Source: CAD feature listing. Evaluate the final solid. Frame: model axes, mm. A direction names the side the tool comes from. Give positions to 0.01 mm unless a question says otherwise; leave off trailing zeros. Write each loop counter-clockwise with the first axis right and the second up, starting at its lowest first coordinate (ties: lowest second). Pieces come first, ordered by that corner, then holes. Notation, with made-up numbers: (49, 43) -> (85, 43) arc R3 ccw to (85, 47) -> close; hole circle Ø11 at (42.5, -1). An arc over 180 degrees is marked (long way). Use one line per item in the form item = value. Start each with the question number.
(1) Cut plane C-C, the plane z = -12. Output: boundary loops of the cut face in (x, y).
(2) Draft query along Y for faces 1 (the face through (0, 6, 2)), 2 (the face through (-22, -0.1, 4.5)), 3 (the face through (-3.233, -1.341, 2.465)). Return one class per face: pulls with the +Y half, pulls with the -Y half, needs draft (parallel to the pull), parting line crosses it, or undercut.
(3) Cut plane A-A, the plane x = -3. Output: boundary loops of the cut face in (y, z).
(4) Set-up query: faces 4 (the face through (15, 0, -7)), 5 (the face through (-16.89, 1.34, -5.08)), 6 (the face through (0, -6, 2)), 7 (the face through (19, 4, -12)). Return all of +Z, -Z, +X, -X, +Y, -Y with unobstructed straight access to the full face (end or side cutting, diameter ignored); none if empty.
(5) Cut plane D-D, the plane z = 1.75. Output: boundary loops of the cut face in (x, y).
(6) Material intervals for line 1 along X through (y, z) = (0, -2.75); line 2 along Y through (x, z) = (0, 3.2); line 3 along X through (y, z) = (2.75, -4.5), sorted ascending. Write a range as from..to.
(7) First-contact query: P1, Ø2.5, axis at x = 19, z = -12.5, coming from the +Y side; P2, Ø4, axis at x = -18, y = -1.5, coming from the -Z side; P3, Ø9, axis at x = -5.5, z = 1.5, coming from the -Y side; P4, Ø6, axis at y = -6.5, z = -3.5, coming from the +X side. Flat tips, straight axial feed; report the tip coordinate or a pass-through.
(8) Cut plane B-B, the plane z = -8.5. Output: boundary loops of the cut face in (x, y), and give its area (3 significant figures).
from build123d import *

# Parameters (mm, degrees)
SKETCH_1_W          = 45
SKETCH_1_H          = 12
EXTRUDE_1_DEPTH     = 5
EXTRUDE_2_DEPTH     = 7.5
SKETCH_9_R          = 3.5
CUT_EXTRUDE_1_DEPTH = 30.382179974
CHAMFER_1_SIZE      = 1


with BuildPart() as part:
    # 草图1 → 凸台-拉伸1 (new body)
    with BuildSketch(Plane.XY):
        Rectangle(SKETCH_1_W, SKETCH_1_H)
    extrude(amount=EXTRUDE_1_DEPTH)

    # 草图4 → 凸台-拉伸2 (add)
    with BuildSketch(Plane(origin=(22.5, 0, 0), x_dir=(0, 0, -1), z_dir=(1, 0, 0))):
        with BuildLine():
            Line((0, 6), (3.364729271, 6))
            ThreePointArc((3.364729271, 6), (4.236286698, 6.038053019), (5.101211047, 6.15192247))
            Line((5.101211047, 6.15192247), (17, 8.25))
            Line((17, 8.25), (17, 6.708203932))
            ThreePointArc((17, 6.708203932), (14.8977866, 5.672023027), (13.255437353, 4))
            Line((13.255437353, 4), (11, 4))
            Line((11, 4), (11, -4))
            Line((11, -4), (13.255437353, -4))
            ThreePointArc((13.255437353, -4), (14.8977866, -5.672023027), (17, -6.708203932))
            Line((17, -6.708203932), (17, -8.25))
            Line((17, -8.25), (5.101211047, -6.15192247))
            ThreePointArc((5.101211047, -6.15192247), (4.236286698, -6.038053019), (3.364729271, -6))
            Line((3.364729271, -6), (0, -6))
            Line((0, -6), (0, 6))
        make_face()
    extrude_2 = extrude(amount=-EXTRUDE_2_DEPTH)

    # 镜向1: 凸台-拉伸2 across plane
    add(extrude_2.mirror(Plane(origin=(0, 0, 0), x_dir=(0, 0, 1), z_dir=(1, 0, 0))))

    # 草图9 → 切除-拉伸1 (cut, through all)
    with BuildSketch(Plane(origin=(0, 0, 0), x_dir=(-1, 0, 0), z_dir=(0, 0, -1))):
        Circle(SKETCH_9_R)
    extrude(amount=-CUT_EXTRUDE_1_DEPTH, mode=Mode.SUBTRACT)

    # 草图12 → M6 螺纹孔1 (revolve, cut)
    with BuildSketch(Plane(origin=(19, 0, -11), x_dir=(0, 1, 0), z_dir=(1, 0, 0))):
        Polygon((0, 0), (0, 13.502151548), (2.5, 12), (2.5, 0), align=None)
    hole_wizard_m6_1 = revolve(axis=Axis((19, 0, -17.35), (0, 0, 1)), mode=Mode.SUBTRACT)

    # 镜向2: M6 螺纹孔1 across plane
    add(hole_wizard_m6_1.mirror(Plane(origin=(0, 0, 0), x_dir=(0, 0, 1), z_dir=(1, 0, 0))), mode=Mode.SUBTRACT)

    # 倒角1
    chamfer_1_edges = [part.edges().sort_by_distance(p)[0] for p in [
        (-22.5, 0, 5),
        (22.5, 0, 5),
    ]]
    chamfer(chamfer_1_edges, length=CHAMFER_1_SIZE)


solid = part.part
Geometry says:
q1.outline = (-22.5, -7.37) -> (-15, -7.37) -> (-15, -4) -> (-22.5, -4) -> close; (-22.5, 4) -> (-15, 4) -> (-15, 7.37) -> (-22.5, 7.37) -> close; (15, -7.37) -> (22.5, -7.37) -> (22.5, -4) -> (15, -4) -> close; (15, 4) -> (22.5, 4) -> (22.5, 7.37) -> (15, 7.37) -> close
q2.face_1 = pulls with the +Y half
q2.face_2 = needs draft
q2.face_3 = undercut
q3.outline = (-6, 0) -> (-1.8, 0) -> (-1.8, 5) -> (-6, 5) -> close; (1.8, 0) -> (6, 0) -> (6, 5) -> (1.8, 5) -> close
q4.face_4 = -Z, +Y, -Y
q4.face_5 = -Z
q4.face_6 = +Z, +X, -X, -Y
q4.face_7 = -Z, +X, -X
q5.outline = (-22.5, -6) -> (22.5, -6) -> (22.5, 6) -> (-22.5, 6) -> close; hole circle Ø2.5 at (-19, 0); hole circle Ø7 at (0, 0); hole circle Ø2.5 at (19, 0)
q6.line_1 = -22.5..-21.5, -16.5..-15, 15..16.5, 21.5..22.5
q6.line_2 = -6..-3.5, 3.5..6
q6.line_3 = -22.5..-15, 15..22.5
q7.P1 = 7.68
q7.P2 = -11
q7.P3 = -6
q7.P4 = 22.5
q8.outline = (-22.5, -6.75) -> (-15, -6.75) -> (-15, 6.75) -> (-22.5, 6.75) -> close; (15, -6.75) -> (22.5, -6.75) -> (22.5, 6.75) -> (15, 6.75) -> close; hole circle Ø5 at (-19, 0); hole circle Ø5 at (19, 0)
q8.area = 163 mm^2
